from build123d import *

# Parameters (mm, degrees)
F0_R     = 2.15265
F0_R_2   = 4.9149
F1_DEPTH = 4.7625
F2_R     = 6.5024
F3_DEPTH = 3.175


with BuildPart() as f1:
    # F0 (on Top) → F1 (new body)
    with BuildSketch(Plane.XY):
        with BuildLine():
            ThreePointArc((9.525, 0), (4.7625, 4.7625), (0, 0))
            Line((0, 0), (0, -79.375))
            ThreePointArc((0, -79.375), (4.7625, -84.1375), (9.525, -79.375))
            Line((9.525, -79.375), (9.525, -49.3649))
            Line((9.525, -49.3649), (60.735159, -49.3649))
            Line((60.735159, -49.3649), (60.735159, -79.375))
            ThreePointArc((60.735159, -79.375), (65.497659, -84.1375), (70.260159, -79.375))
            Line((70.260159, -79.375), (70.260159, 0))
            ThreePointArc((70.260159, 0), (65.497659, 4.7625), (60.735159, 0))
            Line((60.735159, 0), (60.735159, -30.0101))
            Line((60.735159, -30.0101), (9.525, -30.0101))
            Line((9.525, -30.0101), (9.525, 0))
        make_face()
        with Locations((4.7625, -79.375)):
            Circle(F0_R, mode=Mode.SUBTRACT)
        with Locations((65.497659, -79.375)):
            Circle(F0_R, mode=Mode.SUBTRACT)
        with Locations((4.7625, 0)):
            Circle(F0_R, mode=Mode.SUBTRACT)
        with Locations((35.13008, -39.6875)):
            Circle(F0_R_2, mode=Mode.SUBTRACT)
        with Locations((65.497659, 0)):
            Circle(F0_R, mode=Mode.SUBTRACT)
    extrude(amount=F1_DEPTH)

    # F2 (on face) → F3 (cut)
    with BuildSketch(Plane.XY.offset(4.7625)):
        with Locations((35.13008, -39.6875)):
            Circle(F2_R)
    extrude(amount=-F3_DEPTH, mode=Mode.SUBTRACT)


solid = f1.part
The listing builds one solid part. Answer for the finished solid, in the listing's coordinates (mm). A direction names the side the tool comes from. Give positions to 0.01 mm unless a question says otherwise; leave off trailing zeros. Order: outer loops, then holes, each group sorted by start corner. A loop starts at its lowest first (then second) coordinate and runs counter-clockwise, first axis right, second up. Notation, with made-up numbers: (73.5, 28) - (102.5, 28) arc R19 cw to (102.5, 43) - close; hole circle Ø1 at (-27, 89). An arc over 180 degrees is marked (long way). Use one line per item in the form item = value.
1) Find section D-D on x = 59.5. Determine the outline of the cut face in (y, z), and give its area (3 significant figures).
Verdict:
outline = (-49.36, 0) - (-30.01, 0) - (-30.01, 4.76) - (-49.36, 4.76) - close
area = 92.2 mm^2
2) Each of these flat-tipped pins is pushed along its axis until it touches: pin 1 (1.4 mm diameter, centred on x = 31, z = 1.5, fed in from -Y); pin 2 (6 mm diameter, centred on x = 35.13, y = -39.69, fed in from +Z); pin 3 (6.5 mm diameter, centred on x = 37, y = -39, fed in from +Z); pin 4 (1.4 mm diameter, centred on x = 23.5, z = 1.5, fed in from +Y). Where does it stop, or does it pass through?
Verdict:
pin_1 = -49.36
pin_2 = through
pin_3 = 1.59
pin_4 = -30.01
3) Find section C-C on x = 32.5. Determine the outline of the cut face in (y, z), and give its area (3 significant figures).
Verdict:
outline = (-49.36, 0) - (-43.84, 0) - (-43.84, 1.59) - (-45.63, 1.59) - (-45.63, 4.76) - (-49.36, 4.76) - close; (-35.54, 0) - (-30.01, 0) - (-30.01, 4.76) - (-33.74, 4.76) - (-33.74, 1.59) - (-35.54, 1.59) - close
area = 41.2 mm^2
4) Consider probe 1 along X at (y, z) = (-51, 1.55) (3 decimals); probe 2 along Y at (x, z) = (46, 1.3); probe 3 along Y at (x, z) = (64.5, 2.55). Determine where each line is inside the solid, lowest interval first. Write a range as [from, to].
Verdict:
probe_1 = [0, 9.525], [60.735, 70.26]
probe_2 = [-49.36, -30.01]
probe_3 = [-84.03, -81.28], [-77.47, -1.91], [1.91, 4.66]
5) Find section B-B on z = 0.75. Determine the outline of the cut face in (x, y) (1 decimal).
Verdict:
outline = (0, -79.4) arc R4.8 ccw to (9.5, -79.4) - (9.5, -49.4) - (60.7, -49.4) - (60.7, -79.4) arc R4.8 ccw to (70.3, -79.4) - (70.3, 0) arc R4.8 ccw to (60.7, 0) - (60.7, -30) - (9.5, -30) - (9.5, 0) arc R4.8 ccw to (0, 0) - close; hole circle Ø4.3 at (4.8, -79.4); hole circle Ø4.3 at (4.8, 0); hole circle Ø9.8 at (35.1, -39.7); hole circle Ø4.3 at (65.5, -79.4); hole circle Ø4.3 at (65.5, 0)
6) Find section A-A on y = -19. Determine the outline of the cut face in (x, z) (1 decimal).
Verdict:
outline = (0, 0) - (9.5, 0) - (9.5, 4.8) - (0, 4.8) - close; (60.7, 0) - (70.3, 0) - (70.3, 4.8) - (60.7, 4.8) - close
7) For faces 4 (the flat face through (35, -49.365, 2)), 5 (the flat face through (9.525, -15, 2)), 6 (the cylindrical face through (41.137, -42.178, 3.197)), 7 (the cylindrical face through (4.296, -81.476, 2.348)), 8 (the flat face through (40, -46, 4.762)), determine the directions among +Z, -Z, +X, -X, +Y, -Y from which every point of the face is accessible in a straight line to the end or side of a thin tool.
Verdict:
face_4 = +Z, -Z, -Y
face_5 = +Z, -Z, +Y
face_6 = +Z
face_7 = +Z, -Z
face_8 = +Z, +X, -X, +Y, -Y
8) The mould has two halves that part along Y. Classify faces 1 (the cylindrical face through (34.49, -34.814, 0.783)), 2 (the flat face through (60.735, -15, 2)), 3 (the cylindrical face through (65.393, -84.136, 2.348)): released by +Y, released by -Y, zero draft, split by the parting line, or undercut.
Verdict:
face_1 = undercut
face_2 = zero draft
face_3 = released by -Y
